CAD build for the part. Positions are in the model's coordinates, mm. Coordinates: 2 decimals unless noted, no trailing zeros. Answer as CSV lines item,"result". Start each with the question number.
from build123d import *

# Parameters (mm, degrees)
CHAMFER1_SIZE      = 1
FILLET1_R          = 2
SKETCH2_R          = 3
CUT_EXTRUDE1_DEPTH = 114.498898812
CIRPATTERN1_COUNT  = 16


with BuildPart() as part:
    # Sketch1 → Revolve1 (revolve)
    with BuildSketch(Plane.XY, mode=Mode.PRIVATE) as revolve1_sk:
        Polygon((10, 79), (4.656854249, 79), (0, 74.343145751), (-4.656854249, 79), (-10, 79), (-10, 65), (10, 65), align=None)
    revolve(revolve1_sk.sketch.rotate(Axis((-42.067307692, 0, 0), (1, 0, 0)), 90), axis=Axis((-42.067307692, 0, 0), (1, 0, 0)))

    # Chamfer1
    chamfer1_edges = [part.edges().sort_by_distance(p)[0] for p in [
        (10, 0, -65),
        (-10, 0, -65),
    ]]
    chamfer(chamfer1_edges, length=CHAMFER1_SIZE)

    # Fillet1
    fillet1_edges = [part.edges().sort_by_distance(p)[0] for p in [
        (0, 0, -74.343145751),
    ]]
    fillet(fillet1_edges, radius=FILLET1_R)

    # Sketch2 → Cut-Extrude1 (cut, through all)
    with BuildSketch(Plane(origin=(10, 0, 0), x_dir=(0, 0, -1), z_dir=(1, 0, 0))):
        with Locations((0, 72)):
            Circle(SKETCH2_R)
    cut_extrude1 = extrude(amount=-CUT_EXTRUDE1_DEPTH, mode=Mode.SUBTRACT)

    # CirPattern1: Cut-Extrude1 ×16 about axis
    cirpattern1_axis = Axis((0, 0, 0), (1, 0, 0))
    for i in range(1, CIRPATTERN1_COUNT):
        add(cut_extrude1.rotate(cirpattern1_axis, i * 360 / CIRPATTERN1_COUNT), mode=Mode.SUBTRACT)


solid = part.part
Item 1: Wall check: probe 1 along Z at (x, y) = (0.5, 27); probe 2 along Y at (x, z) = (2.25, 0); probe 3 along Z at (x, y) = (-2.5, -30). Give the ranges that are in metal, low to high.
Item 2: Two-plate mould, pull along Y, no slides. Class faces 1 (the face through (-1.617, -22.816, 72.453)), 2 (the face through (10, 64, -17)), 3 (the face through (0.14, 25.832, 64.062)): pulls with the +Y half, pulls with the -Y half, needs draft (parallel to the pull), parting line crosses it, or undercut.
Item 3: Flat gauge pins, fed straight in: pin 1 Ø5 at (y, z) = (-66.52, 27.55) entering from +X; pin 2 Ø1.5 at (x, y) = (3.5, 28.5) entering from +Z; pin 3 Ø8 at (x, y) = (-4.5, 34) entering from -Z; pin 4 Ø2 at (x, y) = (2.5, -61.5) entering from +Z. Where does each tip first touch, or does it go through?
Item 4: Saw through at A-A (z = 0). Count the separate pieces of the cut face and the enclosed holes in it, plus the area to 3 significant figures.
Geometry check:
1,probe 1,"-70.22 to -69.47, -63.57 to -59.13, 59.13 to 63.57, 69.47 to 70.22"
1,probe 2,"-76.59 to -75, -69 to -65, 65 to 69, 75 to 76.59"
1,probe 3,"-70.75 to -68.26, -64.78 to -57.66, 57.66 to 64.78, 68.26 to 70.75"
2,face 1,"parting line crosses it"
2,face 2,"needs draft"
2,face 3,"undercut"
3,pin 1,"through"
3,pin 2,"z = 73.29"
3,pin 3,"z = -73.08"
3,pin 4,"z = 48.16"
4,separate pieces,"4"
4,enclosed holes,"0"
4,area,"276 mm2"
